```python
from build123d import *

# Parameters (mm, degrees)
SKETCH1_R               = 9.7
BOSS_EXTRUDE1_DEPTH     = 3.6
CUT_EXTRUDE1_DEPTH      = 15.182383439
CUT_EXTRUDE1_DEPTH_BACK = 15.182383439
SKETCH2_R               = 0.65
CUT_EXTRUDE2_DEPTH      = 15.182383439
CUT_EXTRUDE2_DEPTH_BACK = 15.182383439
SKETCH3_R               = 3
SKETCH4_R               = 9.7
SKETCH4_R_2             = 3.5
SKETCH4_R_3             = 0.65
CUT_EXTRUDE3_DEPTH      = 0.15


with BuildPart() as part:
    # Sketch1 → Boss-Extrude1 (new body)
    with BuildSketch(Plane(origin=(0, 0, 0), x_dir=(1, 0, 0), z_dir=(0, 1, 0))):
        with Locations(Location((0, 0, 0), (0, 0, 270))):
            Circle(SKETCH1_R)
    extrude(amount=BOSS_EXTRUDE1_DEPTH)

    # Sketch2 → Cut-Extrude1 (cut, two sides: drawn at the far end of the back side and taken through both)
    with BuildSketch(Plane(origin=(0, 3.6, 0), x_dir=(1, 0, 0), z_dir=(0, 1, 0)).offset(-CUT_EXTRUDE1_DEPTH_BACK)):
        with Locations(Location((-6.975, 0, 0), (0, 0, 270))):
            Circle(SKETCH2_R)
        with Locations(Location((-4.932069799, 4.932069799, 0), (0, 0, 270))):
            Circle(SKETCH2_R)
        with Locations(Location((0, 6.975, 0), (0, 0, 270))):
            Circle(SKETCH2_R)
        with Locations(Location((4.932069799, 4.932069799, 0), (0, 0, 270))):
            Circle(SKETCH2_R)
        with Locations(Location((6.975, 0, 0), (0, 0, 270))):
            Circle(SKETCH2_R)
        with Locations(Location((4.932069799, -4.932069799, 0), (0, 0, 270))):
            Circle(SKETCH2_R)
        with Locations(Location((0, -6.975, 0), (0, 0, 270))):
            Circle(SKETCH2_R)
        with Locations(Location((-4.932069799, -4.932069799, 0), (0, 0, 270))):
            Circle(SKETCH2_R)
    extrude(amount=CUT_EXTRUDE1_DEPTH + CUT_EXTRUDE1_DEPTH_BACK, mode=Mode.SUBTRACT)

    # Sketch3 → Cut-Extrude2 (cut, two sides: drawn at the far end of the back side and taken through both)
    with BuildSketch(Plane(origin=(0, 3.6, 0), x_dir=(1, 0, 0), z_dir=(0, 1, 0)).offset(-CUT_EXTRUDE2_DEPTH_BACK)):
        with Locations(Location((0, 0, 0), (0, 0, 270))):
            Circle(SKETCH3_R)
    extrude(amount=CUT_EXTRUDE2_DEPTH + CUT_EXTRUDE2_DEPTH_BACK, mode=Mode.SUBTRACT)

    # Sketch4 → Cut-Extrude3 (cut)
    with BuildSketch(Plane(origin=(0, 3.6, 0), x_dir=(1, 0, 0), z_dir=(0, 1, 0))):
        with Locations(Location((0, 0, 0), (0, 0, 270))):
            Circle(SKETCH4_R)
        with Locations(Location((0, 0, 0), (0, 0, 270))):
            Circle(SKETCH4_R_2, mode=Mode.SUBTRACT)
        with Locations(Location((-6.975, 0, 0), (0, 0, 270))):
            Circle(SKETCH4_R_3, mode=Mode.SUBTRACT)
        with Locations(Location((0, 6.975, 0), (0, 0, 270))):
            Circle(SKETCH4_R_3, mode=Mode.SUBTRACT)
        with Locations(Location((6.975, 0, 0), (0, 0, 270))):
            Circle(SKETCH4_R_3, mode=Mode.SUBTRACT)
        with Locations(Location((0, -6.975, 0), (0, 0, 270))):
            Circle(SKETCH4_R_3, mode=Mode.SUBTRACT)
        with Locations(Location((-4.932069799, -4.932069799, 0), (0, 0, 270))):
            Circle(SKETCH4_R_3, mode=Mode.SUBTRACT)
        with Locations(Location((4.932069799, -4.932069799, 0), (0, 0, 270))):
            Circle(SKETCH4_R_3, mode=Mode.SUBTRACT)
        with Locations(Location((4.932069799, 4.932069799, 0), (0, 0, 270))):
            Circle(SKETCH4_R_3, mode=Mode.SUBTRACT)
        with Locations(Location((-4.932069799, 4.932069799, 0), (0, 0, 270))):
            Circle(SKETCH4_R_3, mode=Mode.SUBTRACT)
    extrude(amount=-CUT_EXTRUDE3_DEPTH, mode=Mode.SUBTRACT)


solid = part.part
```
Could you check a few things on this model? Use its own coordinates, in mm. Round coordinates to 2 decimals unless told otherwise and drop trailing zeros. Write each loop counter-clockwise with the first axis right and the second up, starting at its lowest first coordinate (ties: lowest second). Pieces come first, ordered by that corner, then holes.
(1) Suppose I cut it at C-C on z = -2.25. Write out the boundary of the cut face in (x, y), and give its area (3 significant figures).
Findings below:
outline: (-9.44, 0) - (-1.98, 0) - (-1.98, 3.6) - (-2.68, 3.6) - (-2.68, 3.45) - (-9.44, 3.45) - close; (1.98, 0) - (9.44, 0) - (9.44, 3.45) - (2.68, 3.45) - (2.68, 3.6) - (1.98, 3.6) - close
area: 51.6 mm2
(2) Suppose I cut it at D-D on y = 3.2. State how many separate pieces and enclosed holes the cut face has, and give its area (3 significant figures).
Findings below:
separate pieces: 1
enclosed holes: 9
area: 257 mm2
(3) For pin 1 (1.5 mm diameter, centred on x = 6.975, z = 0, fed in from -Y); pin 2 (2 mm diameter, centred on x = -2, y = 2, fed in from +Z); pin 3 (1.5 mm diameter, centred on x = 0, z = 6.975, fed in from +Y); pin 4 (2 mm diameter, centred on x = -5, y = 1.5, fed in from -Z), each with a flat end and sliding along its axis, tell me the tip position at first contact or that it passes through.
Findings below:
pin 1: stops at y = 0
pin 2: stops at z = 9.65
pin 3: stops at y = 3.45
pin 4: stops at z = -8.84
(4) Suppose I cut it at A-A on z = 0. Write out the boundary of the cut face in (x, y) (3 decimals), and give its area (3 significant figures).
Findings below:
outline: (-9.7, 0) - (-7.625, 0) - (-7.625, 3.45) - (-9.7, 3.45) - close; (-6.325, 0) - (-3, 0) - (-3, 3.6) - (-3.5, 3.6) - (-3.5, 3.45) - (-6.325, 3.45) - close; (3, 0) - (6.325, 0) - (6.325, 3.45) - (3.5, 3.45) - (3.5, 3.6) - (3, 3.6) - close; (7.625, 0) - (9.7, 0) - (9.7, 3.45) - (7.625, 3.45) - close
area: 37.4 mm2
(5) If I drill on probe 1 along X at (y, z) = (1.2, 0) (3 decimals); probe 2 along X at (y, z) = (0.5, 4.5); probe 3 along X at (y, z) = (1.1, -5.25), over which ranges is the centre line in solid material (lowest first)?
Findings below:
probe 1: x = -9.7 to -7.625, -6.325 to -3, 3 to 6.325, 7.625 to 9.7
probe 2: x = -8.59 to -5.42, -4.45 to 4.45, 5.42 to 8.59
probe 3: x = -8.16 to -5.5, -4.37 to 4.37, 5.5 to 8.16
(6) Thinking about a two-plate mould opening in Z: for faces 1 (the face through (-6.33, 1.7, -0.08)), 2 (the face through (2.914, 1.701, 9.252)), 3 (the face through (0, 3.45, 4)), which applies, +Z half, -Z half, draft (parallel to the pull), parting line (faces both ways), or undercut?
Findings below:
face 1: undercut
face 2: parting line
face 3: draft
(7) Suppose I cut it at B-B on x = 0. Write out the boundary of the cut face in (y, z) (3 decimals).
Findings below:
outline: (0, -9.7) - (3.45, -9.7) - (3.45, -7.625) - (0, -7.625) - close; (0, -6.325) - (3.45, -6.325) - (3.45, -3.5) - (3.6, -3.5) - (3.6, -3) - (0, -3) - close; (0, 3) - (3.6, 3) - (3.6, 3.5) - (3.45, 3.5) - (3.45, 6.325) - (0, 6.325) - close; (0, 7.625) - (3.45, 7.625) - (3.45, 9.7) - (0, 9.7) - close
